Source: CAD feature listing. Evaluate the final solid. Frame: model axes, mm. Face numbers are marked on the shaded views. A direction names the side the tool comes from. Give positions to 0.01 mm unless a question says otherwise; leave off trailing zeros. Loops run counter-clockwise (first coordinate to the right, second up) from the corner with the lowest first, then second, coordinate; pieces in that order, holes last. Notation, with made-up numbers: (84.25, -23) -> (130.25, -23) arc R21 ccw to (130.25, 7) -> close; hole circle Ø11 at (24.5, 7.5). An arc over 180 degrees is marked (long way). Return JSON: item names as keys, results as strings. Group by question number.
(1) Pin query (flat end, axial travel): pin 1 (16.5 mm diameter, centred on x = 18, y = 43, fed in from +Z) (3 decimals); pin 2 (5 mm diameter, centred on x = 66, z = 46.5, fed in from +Y); pin 3 (11 mm diameter, centred on y = -20, z = 0.5, fed in from +X) (3 decimals). Return the tip coordinate at first contact, or that it passes through.
(2) Access query for the marked faces 5, 6, 7 and 8. Directions: +Z, -Z, +X, -X, +Y, -Y. A direction counts if a zero-diameter tool reaches every point of the face in a straight line with its end or side. Return the directions, or none.
(3) Cut plane B-B on x = 94.5. Return loops of the section in (y, z) (3 decimals), then the cut area to 3 significant figures.
(4) Draft query along X for the marked faces 1, 2, 3 and 4. Return one class per face: released by +X, released by -X, zero draft, split by the parting line, or undercut.
(5) Ray query, line 1 (Z direction, x = 22, y = -17.5) (3 decimals); line 2 (X direction, y = 47, z = 8.5) (3 decimals); line 3 (Y direction, x = 51, z = 47). Return the intervals inside material, ascending. Write a range as from..to.
(6) Cut plane A-A on z = -4. Return loops of the section in (x, y) (3 decimals).
```python
from build123d import *

# Parameters (mm, degrees)
F1_DEPTH = 63.5
F2_DEPTH = 25.4
F3_DEPTH = 7.9375


with BuildPart() as f1:
    # F0 (on Front) → F1 (new body, symmetric)
    with BuildSketch(Plane.XZ):
        Polygon((-41.275, 9.525), (-41.275, -9.525), (41.275, -9.525), (41.275, 9.525), (22.225, 9.525), align=None)
    extrude(amount=F1_DEPTH, both=True)

    # F0 (on Front) → F2 (join, symmetric)
    with BuildSketch(Plane.XZ):
        with BuildLine():
            Line((22.225, 9.525), (41.275, 9.525))
            Line((41.275, 9.525), (41.275, 26.3144))
            ThreePointArc((41.275, 26.3144), (45.9246798487, 37.5397201513), (57.15, 42.1894))
            Line((57.15, 42.1894), (60.325, 42.1894))
            Line((60.325, 42.1894), (60.325, 61.2394))
            Line((60.325, 61.2394), (57.15, 61.2394))
            add(Edge.make_bspline(
                [(54.4521083612, 61.1350405126), (55.3312639193, 61.1719383272), (56.2302041727, 61.2066578487), (57.15, 61.2394)],
                knots=[0.9818500248, 0.9818500248, 0.9818500248, 0.9818500248, 1, 1, 1, 1], degree=3))
            ThreePointArc((54.4521083612, 61.1350405126), (31.5181888029, 50.0370870265), (22.225, 26.3144))
            Line((22.225, 26.3144), (22.225, 9.525))
        make_face()
        Polygon((60.325, 66.675), (60.325, 61.2394), (60.325, 42.1894), (60.325, 38.1), (111.125, 38.1), (111.125, 66.675), align=None)
    extrude(amount=F2_DEPTH, both=True)

    # F0 (on Front) → F3 (join, symmetric)
    with BuildSketch(Plane.XZ):
        with BuildLine():
            add(Edge.make_bspline(
                [(-41.275, 9.525), (-28.348620981, 29.8197139055), (11.5454759395, 55.3722683758), (33.0508519988, 60.2368381598), (54.4521083612, 61.1350405126)],
                knots=[0, 0, 0, 0, 0.540025743, 0.9818500248, 0.9818500248, 0.9818500248, 0.9818500248], degree=3))
            Line((-41.275, 9.525), (22.225, 9.525))
            Line((22.225, 9.525), (22.225, 26.3144))
            ThreePointArc((22.225, 26.3144), (31.5181888029, 50.0370870265), (54.4521083612, 61.1350405126))
        make_face()
    extrude(amount=F3_DEPTH, both=True)


solid = f1.part
```
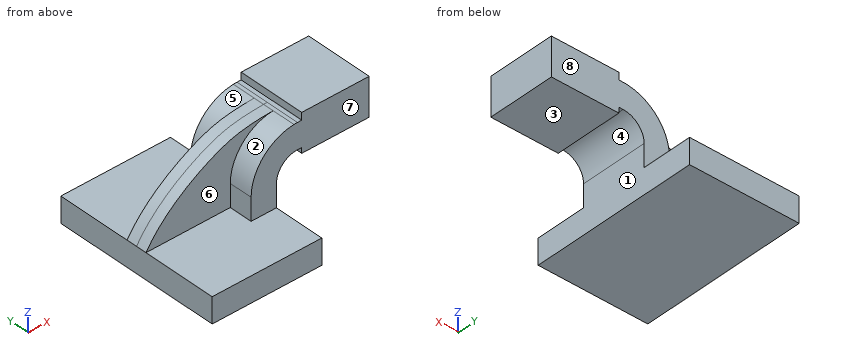
Answers:
{
 "1": {"pin 1": "z = 9.525", "pin 2": "y = 25.4", "pin 3": "x = 41.275"},
 "2": {"face 5": "+Z, -X, +Y", "face 6": "+Z, -X, -Y", "face 7": "+Z, +X, -X, -Y", "face 8": "+Z, +X, -X, +Y"},
 "3": {"outline": "(-25.4, 38.1) -> (25.4, 38.1) -> (25.4, 66.675) -> (-25.4, 66.675) -> close", "area": "1,450 mm²"},
 "4": {"face 1": "released by +X", "face 2": "released by -X", "face 3": "zero draft", "face 4": "undercut"},
 "5": {"line 1": "-9.525..9.525", "line 2": "-41.275..41.275", "line 3": "-25.4..25.4"},
 "6": {"outline": "(-41.275, -63.5) -> (41.275, -63.5) -> (41.275, 63.5) -> (-41.275, 63.5) -> close"}
}
